Study the drawing (mm; zero at the part's minimum x, y, z) and answer. Coordinates: 2 decimals unless noted, no trailing zeros. Order: outer loops, then holes, each group sorted by start corner. A loop starts at its lowest first (then second) coordinate and runs counter-clockwise, first axis right, second up. Notation, with made-up numbers: M 21,-39.75 L 34,-39.75 A16 cw 34,-18.75 Z; hole C 71,1.25 d3. An arc over 180 degrees is marked long. Put each result on its own line as item: value.
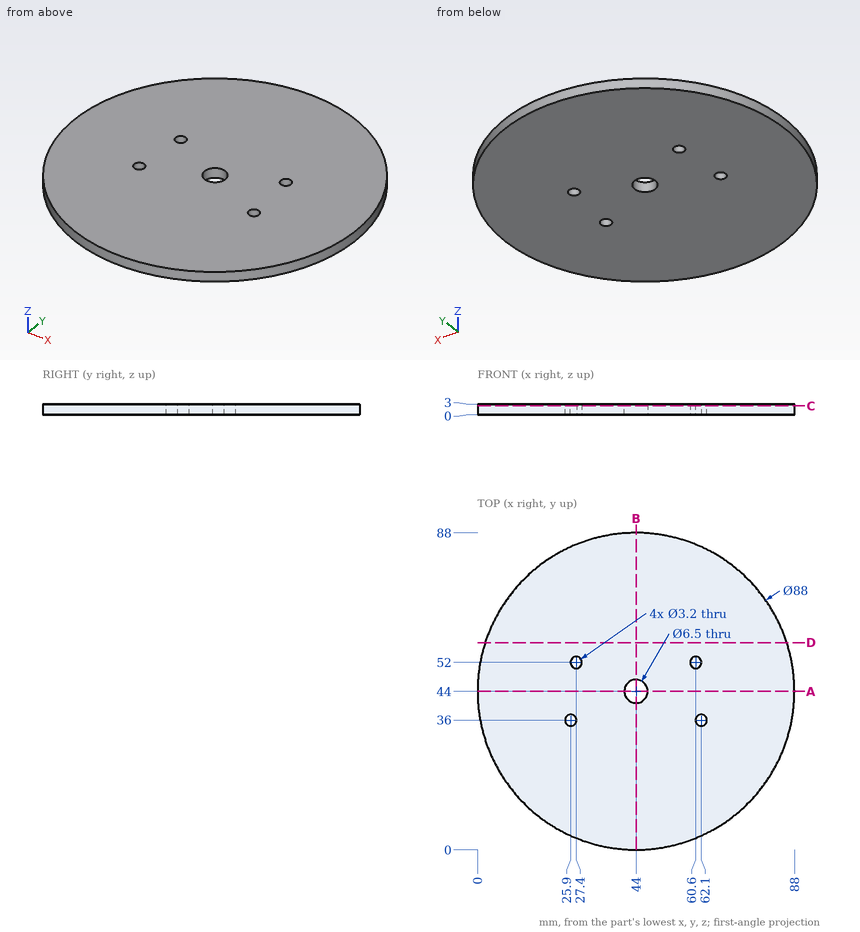
Q1. Consider line 1 along Y through (x, z) = (44, 2.3); line 2 along X through (y, z) = (53, 1.5); line 3 along X through (y, z) = (42, 2.8). Determine where each line is inside the solid, lowest interval first.
Answers below:
line 1: y = 0 to 40.75, 47.25 to 88
line 2: x = 0.93 to 26.15, 28.65 to 59.35, 61.85 to 87.07
line 3: x = 0.05 to 41.44, 46.56 to 87.95
Q2. Find section D-D on y = 57.5. Write down the section's boundary in (x, z).
Answers below:
outline: M 2.12,0 L 85.88,0 L 85.88,3 L 2.12,3 Z
Q3. Find section A-A on y = 44. Write down the section's boundary in (x, z), plus the area to 4 significant figures.
Answers below:
outline: M 0,0 L 40.75,0 L 40.75,3 L 0,3 Z; M 47.25,0 L 88,0 L 88,3 L 47.25,3 Z
area: 244.5 mm^2
Q4. Given pin 1 (4 mm diameter, centred on x = 25.9, y = 36, fed in from -Z); pin 2 (1 mm diameter, centred on y = 26.5, z = 0.5, fed in from +X); pin 3 (3 mm diameter, centred on x = 60.6, y = 52, fed in from +Z); pin 4 (1 mm diameter, centred on x = 71, z = 0.5, fed in from +Y), each flat-ended and moving along its own axis, determine where each tip first touches the part or whether it passes through.
Answers below:
pin 1: stops at z = 0
pin 2: stops at x = 84.58
pin 3: passes through
pin 4: stops at y = 79.12
Q5. Find section C-C on z = 2.5. Write down the section's boundary in (x, y), plus the area to 3 significant figures.
Answers below:
outline: C 44,44 d88; hole C 25.9,36 d3.2; hole C 27.4,52 d3.2; hole C 44,44 d6.5; hole C 60.6,52 d3.2; hole C 62.1,36 d3.2
area: 6,020 mm^2
